Design review of the part shown in the three views and the two pictorial views. Dimensions are in mm from the part's minimum x, y and z. Give positions to 0.01 mm unless a question says otherwise; leave off trailing zeros. Loops run counter-clockwise (first coordinate to the right, second up) from the corner with the lowest first, then second, coordinate; pieces in that order, holes last. Notation, with made-up numbers: (-27.5, 87) - (22.5, 87) arc R14 ccw to (22.5, 96) - close; hole circle Ø2 at (-24, 16). An arc over 180 degrees is marked (long way). Answer as a JSON object with one key per item and string values.
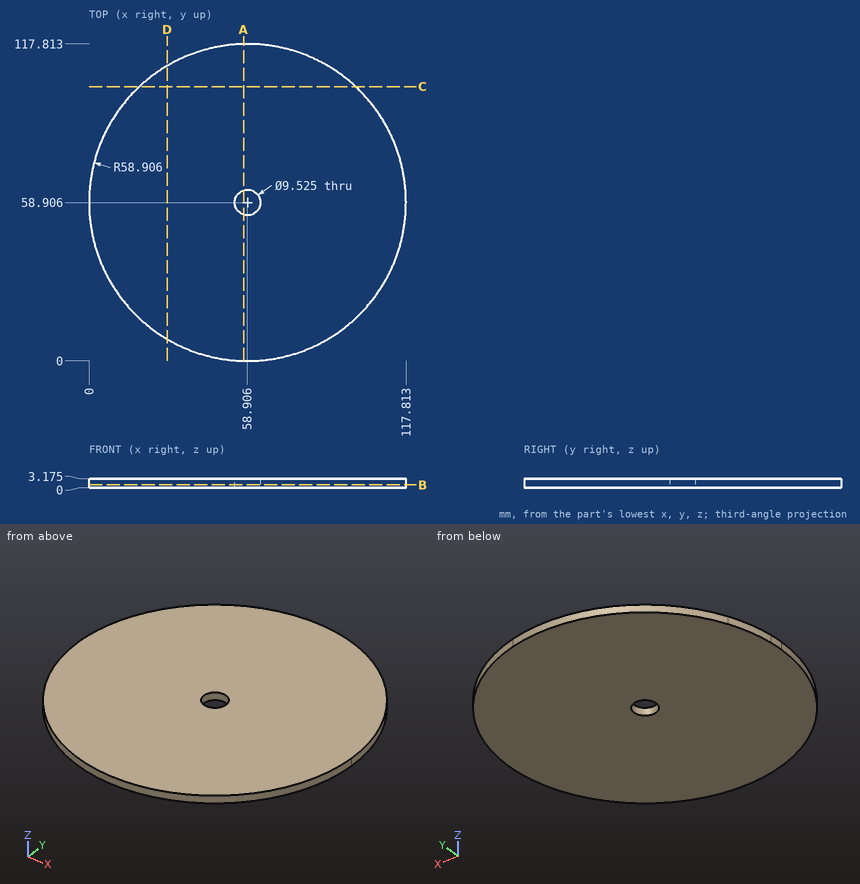
Q1. Consider section A-A, the plane x = 57.5. State the section outline as (y, z) points (1 decimal), plus the area to 3 significant figures.
Results:
{"outline": "(0, 0) - (54.4, 0) - (54.4, 3.2) - (0, 3.2) - close; (63.5, 0) - (117.8, 0) - (117.8, 3.2) - (63.5, 3.2) - close", "area": "345 mm^2"}
Q2. Consider section D-D, the plane x = 29. State the section outline as (y, z) points (1 decimal).
Results:
{"outline": "(8.2, 0) - (109.7, 0) - (109.7, 3.2) - (8.2, 3.2) - close"}
Q3. Consider section C-C, the plane y = 102. State the section outline as (x, z) points (1 decimal).
Results:
{"outline": "(18.7, 0) - (99.1, 0) - (99.1, 3.2) - (18.7, 3.2) - close"}
Q4. To check wall thickness, follow probe 1 along Y at (x, z) = (55, 2.55) (1 decimal); probe 2 along X at (y, z) = (31, 2); probe 3 along X at (y, z) = (11, 1.75) (1 decimal). State the ranges of each line that lie inside material, in increasing order. Write a range as [from, to].
Results:
{"probe 1": "y = [0.1, 56.2], [61.6, 117.7]", "probe 2": "x = [7.03, 110.78]", "probe 3": "x = [24.6, 93.2]"}
Q5. Clearance check with a flat-ended pin moving along its axis: pin 1 Ø1.5 at (x, z) = (25, 2) entering from +Y (1 decimal). State where the tip first meets the part, or that it passes through.
Results:
{"pin 1": "stops at y = 107.6"}
Q6. Consider section B-B, the plane z = 1. State the section outline as (x, y) points (1 decimal).
Results:
{"outline": "circle Ø117.8 at (58.9, 58.9); hole circle Ø9.5 at (58.9, 58.9)"}
